Verification items for the finished model (mm, model axes). Face numbers are marked on the shaded views. A direction names the side the tool comes from. Coordinates: 2 decimals unless noted, no trailing zeros. Loops run counter-clockwise (first coordinate to the right, second up) from the corner with the lowest first, then second, coordinate; pieces in that order, holes last. Notation, with made-up numbers: (-5, 79.5) - (41, 79.5) arc R18 ccw to (41, 98.5) - close; hole circle Ø5 at (63, 82.5). An arc over 180 degrees is marked (long way). Answer as CSV lines item,"result". Start each with the question number.
1. Set-up check for the marked faces 4, 5 and 6: record each of +Z, -Z, +X, -X, +Y, -Y from which the full face is reachable in a straight line by a thin tool's end or side.
2. Material ranges on line 1 (Z direction, x = 7, y = 31.75); line 2 (Y direction, x = 32.3, z = -31.75) (3 decimals); line 3 (X direction, y = 20, z = -25) (1 decimal), recorded low to high. Write a range as [from, to].
3. Gauge pin test, flat ends, axial feed: P1, Ø5.5, axis at y = 31.75, z = -31.75, coming from the +X side; P2, Ø5, axis at x = 13, y = 33, coming from the +Z side; P3, Ø8, axis at x = 32.5, z = -15, coming from the +Y side; P4, Ø12, axis at x = 30, y = 20, coming from the +Z side. Record the tip position at first contact, or that the pin passes through.
4. Cross-section at C-C (x = 7). Enter the section's corners in (y, z).
5. Cross-section at B-B (y = 14). Enter the section's corners in (x, z) (1 decimal), plus the area to 3 significant figures.
6. Cross-section at D-D (z = -33). State how many separate pieces and enclosed holes the cut face has, plus the area to 3 significant figures.
7. Release check for a two-part mould opening along Y. For the marked faces 1, 2 and 3 record: pulls with the +Y half, pulls with the -Y half, needs draft (parallel to the pull), parting line crosses it, or undercut.
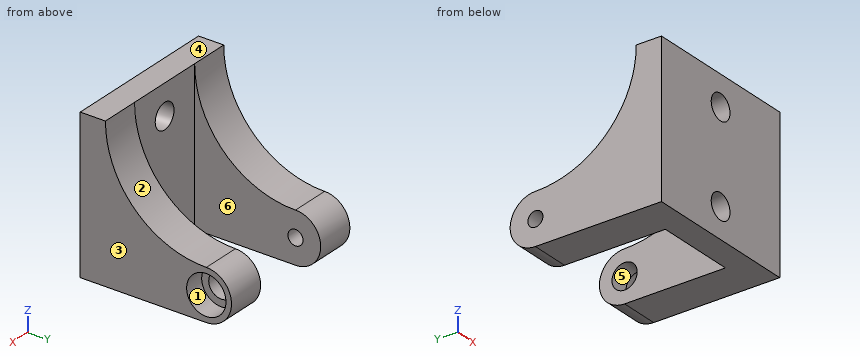
```python
from build123d import *

# Parameters (mm, degrees)
EXTRUDE3_DEPTH                 = 40.005
SKETCH6_W                      = 20.32
SKETCH6_H                      = 42.20483691
EXTRUDE_SLOT_DEPTH             = 39.1
SKETCH8_R                      = 3.175
EXTRUDE_SHOULDER_THROUGH_DEPTH = 9.8425
SKETCH9_R                      = 4.953
EXTRUDE_CNTR_BORE_DEPTH        = 5.08
F_10_24_TAPPED_HOLE1_D         = 3.7973
F_10_24_TAPPED_HOLE1_DEPTH     = 12.827
F_10_24_TAPPED_HOLE1_TIP       = 1.140824014
SKETCH13_R                     = 3.175
EXTRUDE7_DEPTH                 = 39.1


with BuildPart() as part:
    # Sketch5 → Extrude3 (new body)
    with BuildSketch(Plane(origin=(0, 0, 0), x_dir=(0, 0, -1), z_dir=(1, 0, 0))):
        with BuildLine():
            Line((0, 0), (38.1, 0))
            Line((38.1, 0), (38.1, 31.75))
            ThreePointArc((38.1, 31.75), (31.75, 38.1), (25.4, 31.75))
            ThreePointArc((25.4, 31.75), (17.960512242, 13.789487758), (0, 6.35))
            Line((0, 6.35), (0, 0))
        make_face()
    extrude(amount=EXTRUDE3_DEPTH)

    # Sketch6 → Extrude - Slot (cut, through all)
    with BuildSketch(Plane(origin=(0, 0, -38.1), x_dir=(-1, 0, 0), z_dir=(0, 0, -1))):
        with Locations((-20.0025, 27.452418455)):
            Rectangle(SKETCH6_W, SKETCH6_H)
    extrude(amount=-EXTRUDE_SLOT_DEPTH, mode=Mode.SUBTRACT)

    # Sketch8 → Extrude - shoulder through (cut)
    with BuildSketch(Plane(origin=(40.005, 0, 0), x_dir=(0, 0, -1), z_dir=(1, 0, 0))):
        with Locations((31.75, 31.75)):
            Circle(SKETCH8_R)
    extrude(amount=-EXTRUDE_SHOULDER_THROUGH_DEPTH, mode=Mode.SUBTRACT)

    # Sketch9 → Extrude - cntr bore (cut)
    with BuildSketch(Plane(origin=(40.005, 0, 0), x_dir=(0, 0, -1), z_dir=(1, 0, 0))):
        with Locations((31.75, 31.75)):
            Circle(SKETCH9_R)
    extrude(amount=-EXTRUDE_CNTR_BORE_DEPTH, mode=Mode.SUBTRACT)

    # #10-24 Tapped Hole1
    with Locations(Plane(origin=(0, 31.75, -31.75), x_dir=(0, 0, -1), z_dir=(-1, 0, 0))):
        with Locations((0, 0)):
            Hole(F_10_24_TAPPED_HOLE1_D / 2, depth=F_10_24_TAPPED_HOLE1_DEPTH)
            with Locations((0, 0, -(F_10_24_TAPPED_HOLE1_DEPTH + F_10_24_TAPPED_HOLE1_TIP / 2))):  # 118° drill point
                Cone(0, F_10_24_TAPPED_HOLE1_D / 2, F_10_24_TAPPED_HOLE1_TIP, mode=Mode.SUBTRACT)

    # Sketch13 → Extrude7 (cut, through all)
    with BuildSketch(Plane.XZ):
        with Locations((20.0025, -7.62)):
            Circle(SKETCH13_R)
        with Locations((20.0025, -30.48)):
            Circle(SKETCH13_R)
    extrude(amount=-EXTRUDE7_DEPTH, mode=Mode.SUBTRACT)


solid = part.part
```
Values follow:
1,face 4,"+Z, +X, -X, +Y, -Y"
1,face 5,"+X"
1,face 6,"+Z, -Z, +Y"
2,line 1,"z = [-38.1, -33.65], [-29.85, -25.4]"
2,line 2,"y = [0, 28.575], [34.925, 38.1]"
2,line 3,"x = [0, 9.8], [30.2, 40]"
3,P1,"stops at x = 9.84"
3,P2,"passes through"
3,P3,"stops at y = 14.89"
3,P4,"stops at z = -18.17"
4,outline,"(0, -38.1) - (31.75, -38.1) arc R6.35 ccw to (31.75, -25.4) arc R25.4 cw to (6.35, 0) - (0, 0) - close; hole circle Ø3.8 at (31.75, -31.75)"
5,outline,"(0, -38.1) - (9.8, -38.1) - (9.8, -18.2) - (0, -18.2) - close; (30.2, -38.1) - (40, -38.1) - (40, -18.2) - (30.2, -18.2) - close"
5,area,"392 mm²"
6,separate pieces,"4"
6,enclosed holes,"0"
6,area,"747 mm²"
7,face 1,"undercut"
7,face 2,"pulls with the +Y half"
7,face 3,"needs draft"
